from build123d import *

# Parameters (mm, degrees)
ESBO_O1_R                = 5
RESSALTO_EXTRUS_O1_DEPTH = 1
ESBO_O3_R                = 5
RESSALTO_EXTRUS_O3_DEPTH = 15
CORTE_EXTRUS_O2_START    = -15
ESBO_O4_R                = 4.75
CORTE_EXTRUS_O2_DEPTH    = 15
ESBO_O5_R                = 5
RESSALTO_EXTRUS_O4_DEPTH = 1
ESBO_O6_W                = 1
ESBO_O6_H                = 5
CORTE_EXTRUS_O3_DEPTH    = 1


with BuildPart() as part:
    # Esboço1 → Ressalto-extrusão1 (new body)
    with BuildSketch(Plane(origin=(0, 0, 0), x_dir=(1, 0, 0), z_dir=(0, 1, 0))):
        with Locations(Location((0, 0, 0), (0, 0, 270))):
            Circle(ESBO_O1_R)
    extrude(amount=RESSALTO_EXTRUS_O1_DEPTH)

    # Esboço3 → Ressalto-extrusão3 (add)
    with BuildSketch(Plane(origin=(0, 0.5, 0), x_dir=(1, 0, 0), z_dir=(0, 1, 0))):
        with Locations(Location((0, 0, 0), (0, 0, 270))):
            Circle(ESBO_O3_R)
    extrude(amount=RESSALTO_EXTRUS_O3_DEPTH)

    # Esboço4 → Corte-extrusão2 (cut)
    with BuildSketch(Plane(origin=(0, 15.5, 0), x_dir=(1, 0, 0), z_dir=(0, 1, 0)).offset(CORTE_EXTRUS_O2_START)):
        with Locations(Location((0, 0, 0), (0, 0, 270))):
            Circle(ESBO_O4_R)
    extrude(amount=CORTE_EXTRUS_O2_DEPTH, mode=Mode.SUBTRACT)

    # Esboço5 → Ressalto-extrusão4 (add)
    with BuildSketch(Plane(origin=(0, 15.5, 0), x_dir=(1, 0, 0), z_dir=(0, 1, 0))):
        with Locations(Location((0, 0, 0), (0, 0, 270))):
            Circle(ESBO_O5_R)
    extrude(amount=RESSALTO_EXTRUS_O4_DEPTH)

    # Esboço6 → Corte-extrusão3 (cut)
    with BuildSketch(Plane(origin=(0, 16.5, 0), x_dir=(1, 0, 0), z_dir=(0, 1, 0))):
        Rectangle(ESBO_O6_W, ESBO_O6_H)
    extrude(amount=-CORTE_EXTRUS_O3_DEPTH, mode=Mode.SUBTRACT)


solid = part.part
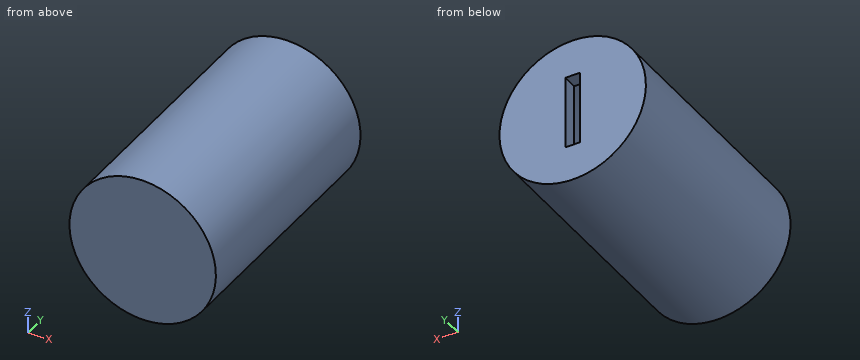
Design review of the part built by this model. Coordinates are the model's own, in mm. Coordinates: 2 decimals unless noted, no trailing zeros. Loops run counter-clockwise (first coordinate to the right, second up) from the corner with the lowest first, then second, coordinate; pieces in that order, holes last. Notation, with made-up numbers: M -16,9 L -12,9 A24 ccw -12,37 Z; hole C 71,45 d8. An arc over 180 degrees is marked long. Use one line per item in the form item = value.
(1) Clearance check with flat-ended pins moving along their axes: P1, Ø0.8, axis at y = 16, z = -1, coming from the -X side; P2, Ø1.5, axis at x = -2, y = 6, coming from the +Z side; P3, Ø3, axis at x = 2, y = 13.5, coming from the +Z side. State where each tip first meets the part, or that it passes through.
Return value:
P1 = -4.96
P2 = 4.84
P3 = 4.97
(2) Consider section C-C (x = -1.5). Write out the cut boundary in (y, z), and give its area (3 significant figures).
Return value:
outline = M 0,-4.77 L 16.5,-4.77 L 16.5,4.77 L 0,4.77 Z; hole M 0.5,-4.51 L 15.5,-4.51 L 15.5,4.51 L 0.5,4.51 Z
area = 22.2 mm2
(3) Consider section D-D (y = 13). Write out the cut boundary in (x, z), and give its area (3 significant figures).
Return value:
outline = C 0,0 d10; hole C 0,0 d9.5
area = 7.66 mm2
(4) Consider section A-A (x = 0). Write out the cut boundary in (y, z), and give its area (3 significant figures).
Return value:
outline = M 0,-5 L 16.5,-5 L 16.5,-2.5 L 15.5,-2.5 L 15.5,-4.75 L 0.5,-4.75 L 0.5,4.75 L 15.5,4.75 L 15.5,2.5 L 16.5,2.5 L 16.5,5 L 0,5 Z
area = 17.5 mm2
(5) For line 1 along Y through (x, z) = (1, -1.25); line 2 along X through (y, z) = (11, 0); line 3 along X through (y, z) = (9.25, 0.75), list the stretches that pass through material, from the lowest coordinate up. Write a range as from..to.
Return value:
line_1 = 0..0.5, 15.5..16.5
line_2 = -5..-4.75, 4.75..5
line_3 = -4.94..-4.69, 4.69..4.94
(6) Consider section B-B (z = -2.75). Write out the cut boundary in (x, y), and give its area (3 significant figures).
Return value:
outline = M -4.18,0 L 4.18,0 L 4.18,16.5 L -4.18,16.5 Z; hole M -3.87,0.5 L 3.87,0.5 L 3.87,15.5 L -3.87,15.5 Z
area = 21.6 mm2
